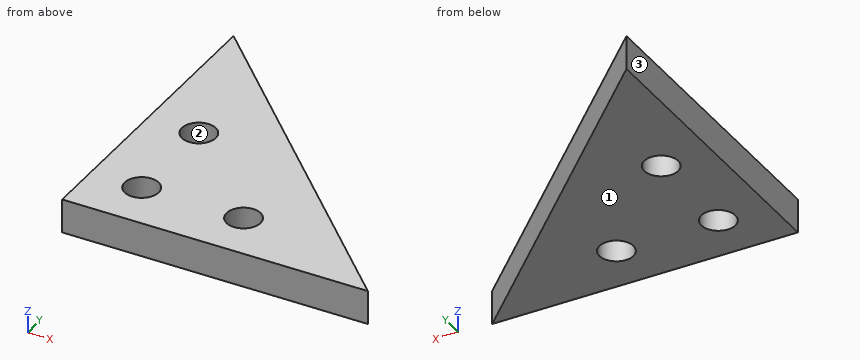
```python
from build123d import *

# Parameters (mm, degrees)
MODEL_R                 = 1.5
SALIENTE_EXTRUIR1_DEPTH = 3


with BuildPart() as part:
    # Model → Saliente-Extruir1 (new body)
    with BuildSketch(Plane.XY):
        Polygon((-105.943383637, 105.556539338), (-105.943383637, 78.556539338), (-78.943383637, 78.556539338), align=None)
        with Locations((-101.443383637, 92.056539338)):
            Circle(MODEL_R, mode=Mode.SUBTRACT)
        with Locations((-101.443383637, 83.056539338)):
            Circle(MODEL_R, mode=Mode.SUBTRACT)
        with Locations((-92.443383637, 83.056539338)):
            Circle(MODEL_R, mode=Mode.SUBTRACT)
    extrude(amount=SALIENTE_EXTRUIR1_DEPTH)


solid = part.part
```
Input: part model. Units: mm. Frame: model coordinates. Face numbers are marked on the shaded views. Coordinates: 2 decimals unless noted, no trailing zeros. Write each loop counter-clockwise with the first axis right and the second up, starting at its lowest first coordinate (ties: lowest second). Pieces come first, ordered by that corner, then holes.
1) Pin query (flat end, axial travel): pin 1 Ø1.8 at (x, y) = (-101.44, 92.06) entering from -Z; pin 2 Ø12 at (x, y) = (-91.5, 92) entering from -Z; pin 3 Ø1 at (x, z) = (-90.5, 2) entering from +Y. Return the tip coordinate at first contact, or that it passes through.
2) Mould query, pull axis X, two halves, no side actions, for the marked faces 1, 2 and 3. Classes: pulls with the +X half, pulls with the -X half, needs draft (parallel to the pull), parting line crosses it, or undercut.
3) Section C-C on z = 1.05. Output: boundary loops of the cut face in (x, y), and give its area (3 significant figures).
4) Section A-A on x = -101.25. Output: boundary loops of the cut face in (y, z), and give its area (3 significant figures).
5) Section D-D on y = 91.5. Output: boundary loops of the cut face in (x, z), and give its area (3 significant figures).
6) Material intervals for line 1 along Y through (x, z) = (-101.75, 0.8); line 2 along X through (y, z) = (82, 0.7); line 3 along Y through (x, z) = (-102, 0.3), sorted ascending.
7) Section B-B on y = 83.5. Output: boundary loops of the cut face in (x, z).
Check result:
1. pin 1: passes through
1. pin 2: stops at z = 0
1. pin 3: stops at y = 90.61
2. face 1: needs draft
2. face 2: undercut
2. face 3: pulls with the -X half
3. outline: (-105.94, 78.56) - (-78.94, 78.56) - (-105.94, 105.56) - close; hole circle Ø3 at (-101.44, 83.06); hole circle Ø3 at (-101.44, 92.06); hole circle Ø3 at (-92.44, 83.06)
3. area: 343 mm2
4. outline: (78.56, 0) - (81.57, 0) - (81.57, 3) - (78.56, 3) - close; (84.54, 0) - (90.57, 0) - (90.57, 3) - (84.54, 3) - close; (93.54, 0) - (100.86, 0) - (100.86, 3) - (93.54, 3) - close
4. area: 49.1 mm2
5. outline: (-105.94, 0) - (-102.84, 0) - (-102.84, 3) - (-105.94, 3) - close; (-100.05, 0) - (-91.89, 0) - (-91.89, 3) - (-100.05, 3) - close
5. area: 33.8 mm2
6. line 1: y = 78.56 to 81.59, 84.52 to 90.59, 93.52 to 101.36
6. line 2: x = -105.94 to -102.51, -100.38 to -93.51, -91.38 to -82.39
6. line 3: y = 78.56 to 81.66, 84.45 to 90.66, 93.45 to 101.61
7. outline: (-105.94, 0) - (-102.88, 0) - (-102.88, 3) - (-105.94, 3) - close; (-100.01, 0) - (-93.88, 0) - (-93.88, 3) - (-100.01, 3) - close; (-91.01, 0) - (-83.89, 0) - (-83.89, 3) - (-91.01, 3) - close
